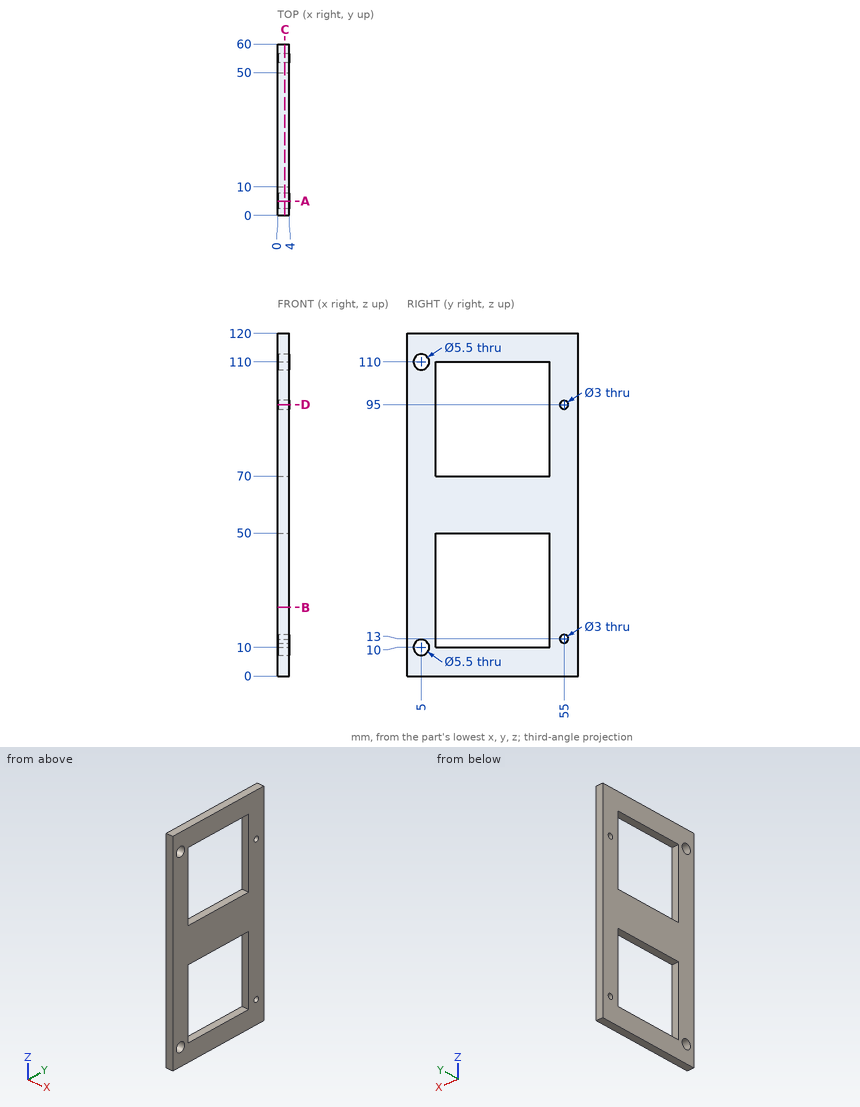
Could you check a few things on this drawing? It's one solid part, dimensions in mm from its lowest x, y, z. Coordinates: 2 decimals unless noted, no trailing zeros. Order: outer loops, then holes, each group sorted by start corner. A loop starts at its lowest first (then second) coordinate and runs counter-clockwise, first axis right, second up. Notation, with made-up numbers: (13, 63) - (27, 63) arc R27 ccw to (27, 101) - close; hole circle Ø7 at (2, 49). An arc over 180 degrees is marked (long way). One line per question, with ' | ' between items. Start each with the question number.
1. Please list where these lines run through material, in increasing order: line 1 along Z through (x, y) = (2.4, 37); line 2 along Y through (x, z) = (1.8, 95); line 3 along Y through (x, z) = (1.3, 22). Write a range as [from, to].
2. If we section it at B-B (z = 24): Write out the boundary of the cut face in (x, y), and give its area (3 significant figures).
3. If we section it at D-D (z = 95): Write out the boundary of the cut face in (x, y).
4. If we section it at A-A (y = 5): Write out the boundary of the cut face in (x, z), and give its area (3 significant figures).
5. If we section it at C-C (x = 2.5): Write out the boundary of the cut face in (y, z).
6. I'm going to push flat-ended pins straight in: pin 1 Ø2.5 at (y, z) = (55, 13) entering from -X; pin 2 Ø6.5 at (y, z) = (5, 10) entering from +X. Where does each tip first touch, or does it pass through?
Model answer:
1) line 1: z = [0, 10], [50, 70], [110, 120] | line 2: y = [0, 10], [50, 53.5], [56.5, 60] | line 3: y = [0, 10], [50, 60]
2) outline: (0, 0) - (4, 0) - (4, 10) - (0, 10) - close; (0, 50) - (4, 50) - (4, 60) - (0, 60) - close | area: 80.0 mm²
3) outline: (0, 0) - (4, 0) - (4, 10) - (0, 10) - close; (0, 50) - (4, 50) - (4, 53.5) - (0, 53.5) - close; (0, 56.5) - (4, 56.5) - (4, 60) - (0, 60) - close
4) outline: (0, 0) - (4, 0) - (4, 7.25) - (0, 7.25) - close; (0, 12.75) - (4, 12.75) - (4, 107.25) - (0, 107.25) - close; (0, 112.75) - (4, 112.75) - (4, 120) - (0, 120) - close | area: 436 mm²
5) outline: (0, 0) - (60, 0) - (60, 120) - (0, 120) - close; hole circle Ø5.5 at (5, 10); hole circle Ø5.5 at (5, 110); hole (10, 10) - (50, 10) - (50, 50) - (10, 50) - close; hole (10, 70) - (50, 70) - (50, 110) - (10, 110) - close; hole circle Ø3 at (55, 13); hole circle Ø3 at (55, 95)
6) pin 1: passes through | pin 2: stops at x = 4
